Work out the finished part from the listing and answer in its coordinate system (mm). A direction names the side the tool comes from. Round coordinates to 2 decimals unless told otherwise and drop trailing zeros. Loops run counter-clockwise (first coordinate to the right, second up) from the corner with the lowest first, then second, coordinate; pieces in that order, holes last. Notation, with made-up numbers: (89.5, 3) -> (126.5, 3) arc R25 cw to (126.5, 30) -> close; hole circle Ø10 at (-37, 87.5). An arc over 180 degrees is marked (long way). Use one line per item in the form item = value.
Autodesk Inventor part; units mm, degrees
ref_plane "YZ Plane" through (0, 0, 0) normal (1, 0, 0) x (0, 1, 0)
ref_plane "XZ Plane" through (0, 0, 0) normal (0, 1, 0) x (-1, 0, 0)
ref_plane "XY Plane" through (0, 0, 0) normal (0, 0, 1) x (1, 0, 0)
sketch "Sketch1" plane through (0, 0, 0) normal (1, 0, 0) x (0, 1, 0)
  circle A0 centre (0, 0) radius 3.175
  circle A1 centre (0, 0) radius 15.875 construction
  line L0 (0, 0) -> (0, 15.875) construction
  circle A2 centre (0, 15.875) radius 1.7526
  circle A3 centre (0, -15.875) radius 1.7526
  line L1 (0, 15.875) -> (0, -15.875) construction
  line L2 (-4.7625, 15.875) -> (-4.7625, -15.875)
  line L3 (4.7625, -15.875) -> (4.7625, 15.875)
  arc A4 (4.7625, 15.875) -> (-4.7625, 15.875) centre (0, 15.875) ccw
  arc A5 (-4.7625, -15.875) -> (4.7625, -15.875) centre (0, -15.875) ccw
  line L4 (1.5875, 15.1324) -> (-1.5875, 15.1324) construction
  line L5 (-1.5875, 15.1324) -> (-1.5875, -15.1324)
  line L6 (-1.5875, -15.1324) -> (1.5875, -15.1324) construction
  line L7 (1.5875, -15.1324) -> (1.5875, 15.1324)
  line L8 (1.5875, 15.1324) -> (-1.5875, -15.1324) construction
  line L9 (-1.5875, 15.1324) -> (1.5875, -15.1324) construction
  circle A6 centre (0, 15.875) radius 4.7625
  circle A7 centre (0, -15.875) radius 4.7625
  point P0 (-4.7625, -15.875)
  point P1 (-1.5875, -11.3849)
  point P2 (-1.5875, -2.7496)
  point P3 (-1.5875, 2.7496)
  point P4 (-1.5875, 11.3849)
  point P5 (1.5875, 11.3849)
  point P6 (1.5875, 2.7496)
  point P7 (1.5875, -2.7496)
  point P8 (1.5875, -11.3849)
  dimension "d1" = 31.75
  dimension "d0" = 6.35
  dimension "d2" = 3.5052
  dimension "d5" = 360
  dimension "d7" = 9.525
  dimension "d8" = 3.175
extrude "Extrusion1" add sketch "Sketch1" along normal blind 1.5875 contours A0 L7 A6 L3 A7 | A0 L5 A6 L7 | L7 A7 L5 A0 | A0 L5 A7 L2 A6 | A6 L5 A2 L7 | L7 A2 L5 A6 A4 | A7 A5 L5 A3 L7 | L7 A3 L5 A7
extrude "Extrusion2" add sketch "Sketch1" along normal blind 6.35 contours A0 L7 A6 L3 A7 | A0 L5 A7 L2 A6
fillet "Fillet1" radius 1.5875 8 edges at (3.9687, 4.7625, 15.875) (3.9687, -4.7625, 15.875) (3.9687, 4.7625, -15.875) (3.9687, -4.7625, -15.875) (3.9687, 1.5875, -11.3849) (3.9687, -1.5875, -11.3849) (3.9687, 1.5875, 11.3849) (3.9687, -1.5875, 11.3849)
fillet "Fillet2" radius 1.5875 4 edges at (3.9687, 1.5875, 2.7496) (3.9687, -1.5875, 2.7496) (3.9687, 1.5875, -2.7496) (3.9687, -1.5875, -2.7496)
properties part number "Pin Slot" material "Aluminum 6061"
(1) Consider L1, parallel to Z at x = 0.65, y = 0 (1 decimal); L2, parallel to Y at x = 0.75, z = 0 (1 decimal); L3, parallel to Z at x = 1.25, y = -1.5. Determine where each line is inside the solid, lowest interval first.
Completed:
L1 = -20.6 to -17.6, -14.1 to -3.2, 3.2 to 14.1, 17.6 to 20.6
L2 = -4.8 to -3.2, 3.2 to 4.8
L3 = -20.4 to -16.78, -14.97 to -2.8, 2.8 to 14.97, 16.78 to 20.4
(2) For faces 1 (the flat face through (4, 1.588, 7)), 2 (the cylindrical face through (4, 3.95, -11.76)), 3 (the cylindrical face through (3.94, 1.73, 2.89)), determine the directions among +Z, -Z, +X, -X, +Y, -Y from which every point of the face is accessible in a straight line to the end or side of a thin tool.
Completed:
face_1 = +Z, -Z, +X
face_2 = -Z, +X
face_3 = +X
(3) Find section B-B, the plane x = 0.5. State how many separate pieces and enclosed holes the cut face has, then the cut area to 3 significant figures.
Completed:
separate_pieces = 1
enclosed_holes = 3
area = 323 mm2
(4) Find section D-D, the plane z = 10. Write down the section's boundary in (x, y).
Completed:
outline = (0, -4.76) -> (6.35, -4.76) -> (6.35, -1.59) -> (1.59, -1.59) -> (1.59, 1.59) -> (6.35, 1.59) -> (6.35, 4.76) -> (0, 4.76) -> close
(5) Find section C-C, the plane y = 0. Write down the section's boundary in (x, z) (1 decimal).
Completed:
outline = (0, -20.6) -> (1.6, -20.6) -> (1.6, -17.6) -> (0, -17.6) -> close; (0, -14.1) -> (1.6, -14.1) -> (1.6, -3.2) -> (0, -3.2) -> close; (0, 3.2) -> (1.6, 3.2) -> (1.6, 14.1) -> (0, 14.1) -> close; (0, 17.6) -> (1.6, 17.6) -> (1.6, 20.6) -> (0, 20.6) -> close
